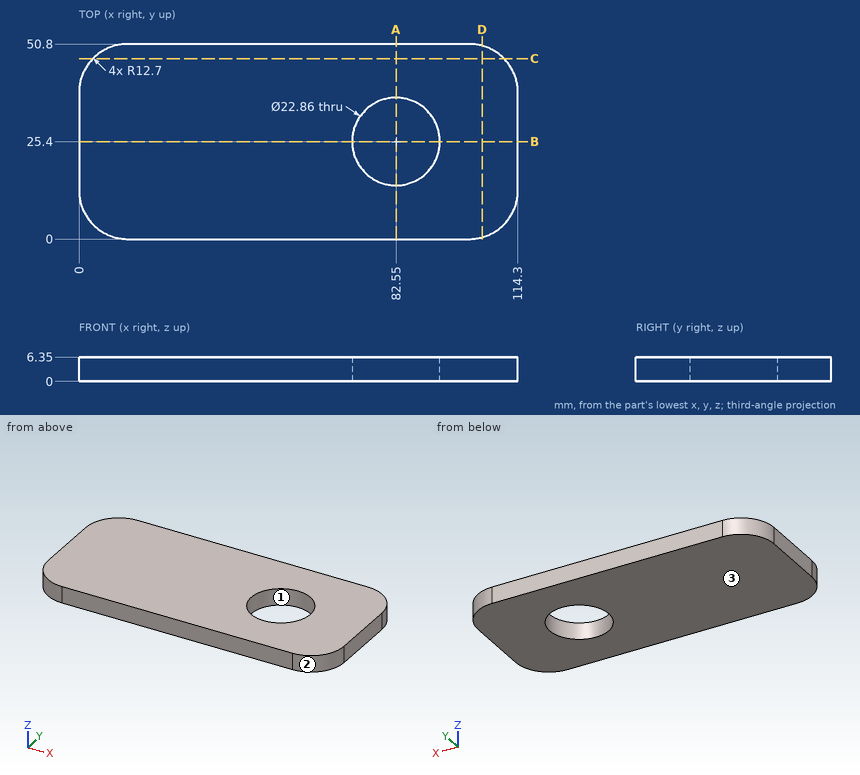
Job drawing, mm, ordinate dimensions from the low corner. One solid piece. Give positions to 0.01 mm unless a question says otherwise; leave off trailing zeros. Loops run counter-clockwise (first coordinate to the right, second up) from the corner with the lowest first, then second, coordinate; pieces in that order, holes last. Notation, with made-up numbers: (55.25, 8.5) -> (78.25, 8.5) arc R6 ccw to (78.25, 14.5) -> close; hole circle Ø2 at (1.25, -16.5). An arc over 180 degrees is marked (long way). Use a Markdown table: item, result. Add a question column.
(1) Wall check: line 1 along Y through (x, z) = (82.55, 3.75); line 2 along X through (y, z) = (25, 6.25); line 3 along X through (y, z) = (15, 4.25). Give the ranges that are in metal, low to high.
(2) Mould opens along X. For the marked faces 1, 2 and 3 say: +X half, -X half, draft (parallel to the pull), parting line (faces both ways), or undercut.
(3) Slice it at B-B on y = 25.4. List the corners of the cut face in (x, z), and give its area (3 significant figures).
(4) Slice it at C-C on y = 47. List the corners of the cut face in (x, z), and give its area (3 significant figures).
(5) Slice it at D-D on x = 105. List the corners of the cut face in (y, z), and give its area (3 significant figures).
(6) Slice it at A-A on x = 82.55. List the corners of the cut face in (y, z), and give its area (3 significant figures).
Filled sheet:
| question | item | result |
|---|---|---|
| 1 | line 1 | 0 to 13.97, 36.83 to 50.8 |
| 1 | line 2 | 0 to 71.13, 93.97 to 114.3 |
| 1 | line 3 | 0 to 77.81, 87.29 to 114.3 |
| 2 | face 1 | undercut |
| 2 | face 2 | +X half |
| 2 | face 3 | draft |
| 3 | outline | (0, 0) -> (71.12, 0) -> (71.12, 6.35) -> (0, 6.35) -> close; (93.98, 0) -> (114.3, 0) -> (114.3, 6.35) -> (93.98, 6.35) -> close |
| 3 | area | 581 mm2 |
| 4 | outline | (3.64, 0) -> (110.66, 0) -> (110.66, 6.35) -> (3.64, 6.35) -> close |
| 4 | area | 680 mm2 |
| 5 | outline | (0.46, 0) -> (50.34, 0) -> (50.34, 6.35) -> (0.46, 6.35) -> close |
| 5 | area | 317 mm2 |
| 6 | outline | (0, 0) -> (13.97, 0) -> (13.97, 6.35) -> (0, 6.35) -> close; (36.83, 0) -> (50.8, 0) -> (50.8, 6.35) -> (36.83, 6.35) -> close |
| 6 | area | 177 mm2 |
